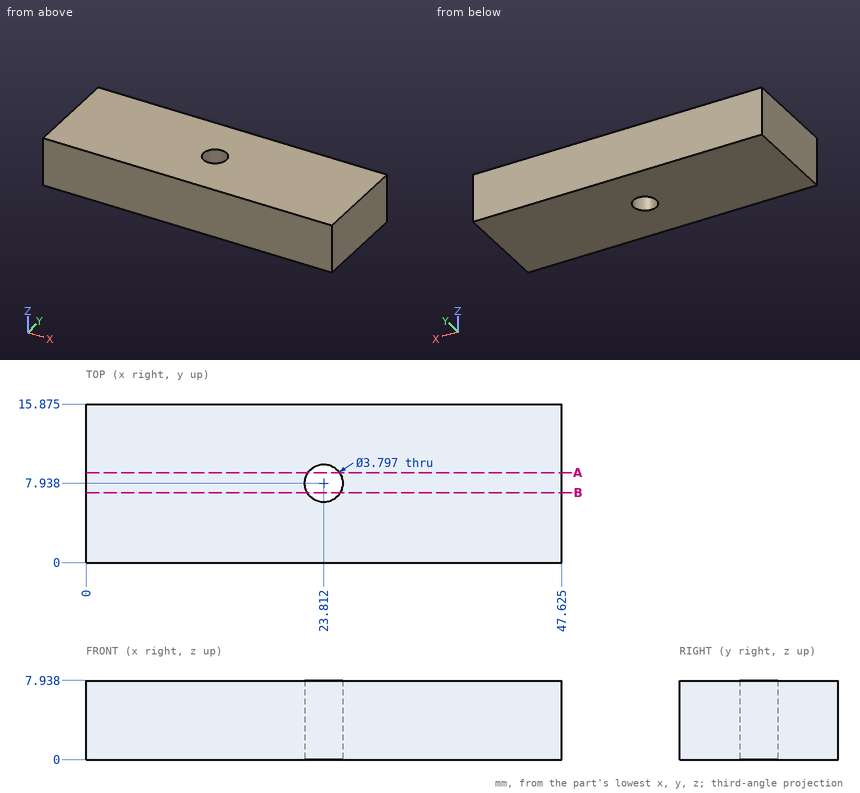
Could you check a few things on this drawing? It's one solid part, dimensions in mm from its lowest x, y, z. Give positions to 0.01 mm unless a question says otherwise; leave off trailing zeros. Order: outer loops, then holes, each group sorted by start corner. A loop starts at its lowest first (then second) coordinate and runs counter-clockwise, first axis right, second up.
1. I need wall thicknesses on L1, parallel to Y at x = 24, z = 1.25 (1 decimal); L2, parallel to X at y = 8.25, z = 5.25 (1 decimal). Which ranges of each line are inside material? Lowest first, please.
Answers below:
L1: y = 0 to 6, 9.8 to 15.9
L2: x = 0 to 21.9, 25.7 to 47.6
2. Suppose I cut it at A-A (y = 9). Write out the boundary of the cut face in (x, z) (1 decimal).
Answers below:
outline: (0, 0) - (22.2, 0) - (22.2, 7.9) - (0, 7.9) - close; (25.4, 0) - (47.6, 0) - (47.6, 7.9) - (25.4, 7.9) - close
3. For pin 1 (3 mm diameter, centred on x = 23.81, y = 7.94, fed in from +Z), with a flat end and sliding along its axis, tell me the tip position at first contact or that it passes through.
Answers below:
pin 1: passes through
4. Suppose I cut it at B-B (y = 7). Write out the boundary of the cut face in (x, z) (1 decimal), plus the area to 3 significant figures.
Answers below:
outline: (0, 0) - (22.2, 0) - (22.2, 7.9) - (0, 7.9) - close; (25.5, 0) - (47.6, 0) - (47.6, 7.9) - (25.5, 7.9) - close
area: 352 mm2
